Could you check a few things on this drawing? It's one solid part, dimensions in mm from its lowest x, y, z. Coordinates: 2 decimals unless noted, no trailing zeros. Write each loop counter-clockwise with the first axis right and the second up, starting at its lowest first coordinate (ties: lowest second). Pieces come first, ordered by that corner, then holes.
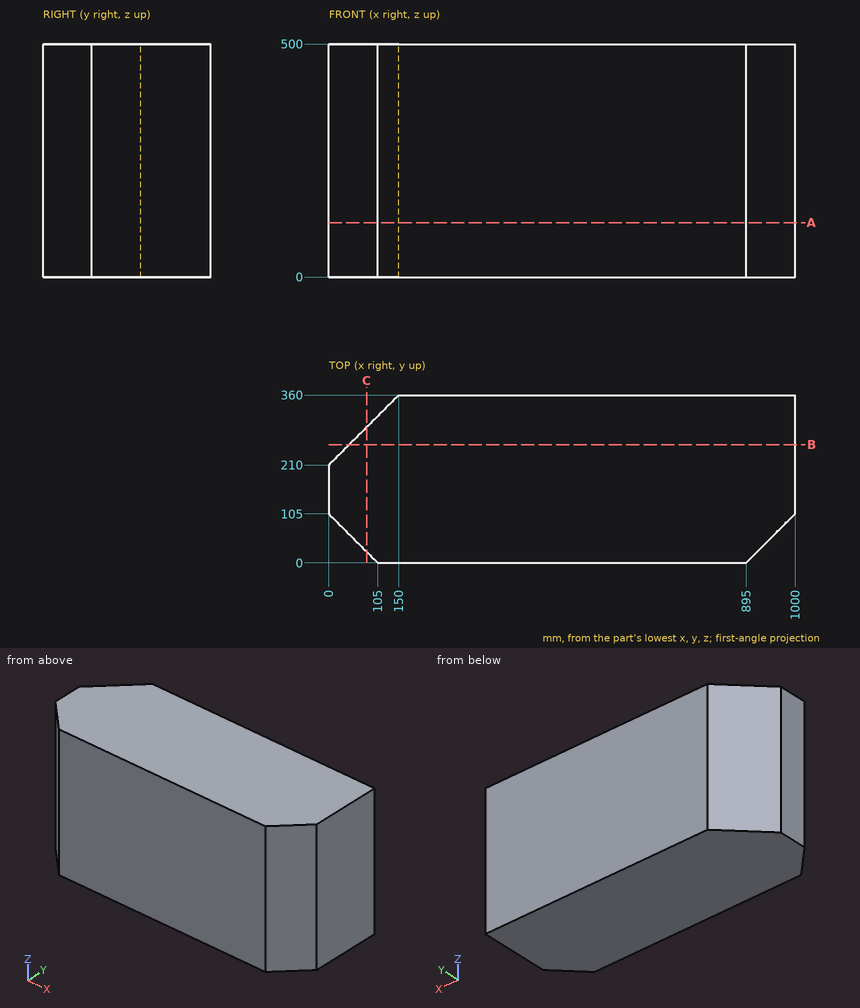
1) Imagine slicing it at A-A on z = 117. Please give me the cut outline in (x, y), then the cut area to 3 significant figures.
Values follow:
outline: (0, 105) - (105, 0) - (895, 0) - (1000, 105) - (1000, 360) - (150, 360) - (0, 210) - close
area: 338,000 mm2
2) I need wall thicknesses on probe 1 along X at (y, z) = (252.5, 298); probe 2 along Y at (x, z) = (107.5, 395.5); probe 3 along Y at (x, z) = (931.5, 161.5). Which ranges of each line are inside material? Lowest first, please.
Values follow:
probe 1: x = 42.5 to 1000
probe 2: y = 0 to 317.5
probe 3: y = 36.5 to 360
3) Imagine slicing it at B-B on y = 253.5. Please give me the cut outline in (x, z), then the cut area to 3 significant figures.
Values follow:
outline: (43.5, 0) - (1000, 0) - (1000, 500) - (43.5, 500) - close
area: 478,000 mm2
4) Imagine slicing it at C-C on x = 81. Please give me the cut outline in (y, z), then the cut area to 4 significant figures.
Values follow:
outline: (24, 0) - (291, 0) - (291, 500) - (24, 500) - close
area: 133,500 mm2
5) Will this pin go through, and if not, where does the flat tip stop? pin 1 (1.5 mm diameter, centred on y = 286, z = 262, fed in from -X).
Values follow:
pin 1: stops at x = 75.25
